Verification items for the finished model (mm, model axes). Round coordinates to 2 decimals unless told otherwise and drop trailing zeros. Loops run counter-clockwise (first coordinate to the right, second up) from the corner with the lowest first, then second, coordinate; pieces in that order, holes last. Notation, with made-up numbers: M 46,64 L 66,64 A20 cw 66,69 Z; hole C 11,12.5 d7. An arc over 180 degrees is marked long. One line per item, written item: value.
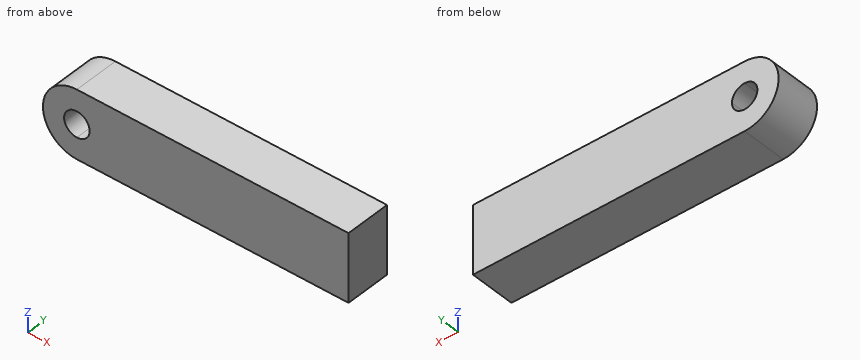
from build123d import *

# Parameters (mm, degrees)
F1_DEPTH = 25.4


with BuildPart() as f1:
    # F0 (on Front) → F1 (new body)
    with BuildSketch(Plane.XZ):
        with BuildLine():
            Line((0, 7.1501), (0, 19.05))
            ThreePointArc((0, 19.05), (-19.05, 0), (0, -19.05))
            Line((0, -19.05), (0, -7.1501))
            ThreePointArc((0, -7.1501), (-7.1501, 0), (0, 7.1501))
        make_face()
        with BuildLine():
            ThreePointArc((0, -19.05), (13.470384, -13.470384), (19.05, 0))
            ThreePointArc((19.05, 0), (13.470384, 13.470384), (0, 19.05))
            Line((0, 19.05), (0, 7.1501))
            ThreePointArc((0, 7.1501), (5.055884, 5.055884), (7.1501, 0))
            ThreePointArc((7.1501, 0), (5.055884, -5.055884), (0, -7.1501))
            Line((0, -7.1501), (0, -19.05))
        make_face()
        with BuildLine():
            ThreePointArc((0, 19.05), (13.470384, 13.470384), (19.05, 0))
            ThreePointArc((19.05, 0), (13.470384, -13.470384), (0, -19.05))
            Line((0, -19.05), (152.4, -19.05))
            Line((152.4, -19.05), (152.4, 19.05))
            Line((152.4, 19.05), (0, 19.05))
        make_face()
    extrude(amount=F1_DEPTH)


solid = f1.part
(1) Depth check by flat-ended pin: pin 1 Ø1.5 at (y, z) = (-18, -0.5) entering from -X. Enter the tip coordinate at first touch or a pass-through.
Completed:
pin 1: stops at x = -19.05
(2) Sectioned sample at C-C on z = -15. Enter the section's corners in (x, y), and give its area (3 significant figures).
Completed:
outline: M -11.74,-25.4 L 152.4,-25.4 L 152.4,0 L -11.74,0 Z
area: 4,170 mm^2
(3) Thickness scan on L1, parallel to X at y = -12.25, z = -0.5; L2, parallel to Z at x = 0.5, y = -20.25; L3, parallel to Z at x = 2, y = -2. Record the ranges inside material, lowest first. Write a range as from..to.
Completed:
L1: x = -19.04..-7.13, 7.13..152.4
L2: z = -19.05..-7.13, 7.13..19.05
L3: z = -19.05..-6.86, 6.86..19.05
(4) Sectioned sample at A-A on y = -17.75. Enter the section's corners in (x, z).
Completed:
outline: M 0,-19.05 L 152.4,-19.05 L 152.4,19.05 L 0,19.05 A19.05 ccw Z; hole M 0,-7.15 A7.15 ccw 7.15,0 A7.15 ccw long Z
(5) Sectioned sample at D-D on z = 14.5. Enter the section's corners in (x, y).
Completed:
outline: M -12.36,-25.4 L 152.4,-25.4 L 152.4,0 L -12.36,0 Z
(6) Sectioned sample at B-B on z = -2.5. Enter the section's corners in (x, y), and give its area (3 significant figures).
Completed:
outline: M -18.89,-25.4 L -6.7,-25.4 L -6.7,0 L -18.89,0 Z; M 6.7,-25.4 L 152.4,-25.4 L 152.4,0 L 6.7,0 Z
area: 4,010 mm^2
